For this review, take the finished solid that the model builds, in its own axes (mm). Face numbers are marked on the shaded views. A direction names the side the tool comes from. Give positions to 0.01 mm unless a question says otherwise; leave off trailing zeros. Order: outer loops, then holes, each group sorted by start corner. A loop starts at its lowest first (then second) coordinate and runs counter-clockwise, first axis right, second up. Notation, with made-up numbers: (22.25, 35.5) -> (56.25, 35.5) arc R24 cw to (56.25, 69.5) -> close; hole circle Ø4 at (73.25, 56.5). An arc over 180 degrees is marked (long way). Return JSON: item names as keys, results as strings. Group by question number.
1) The part is to be moulded in two halves that separate along X. For the marked faces 1, 2 and 3, say which applies: released by +X, released by -X, zero draft, split by the parting line, or undercut.
2) Add section C-C (x = -12). Give the boundary of the cut face in (y, z), then the cut area to 3 significant figures.
3) To check wall thickness, follow line 1 along X through (y, z) = (-17.5, -8); line 2 along X through (y, z) = (7, -7); line 3 along Z through (x, y) = (12.75, -5.05). State the ranges of each line that lie inside material, in increasing order.
4) Add section A-A (z = -21.5). Give the boundary of the cut face in (x, y).
5) For the marked faces 4, 5, 6 and 7, list the 3-axis set-ups (+Z, -Z, +X, -X, +Y, -Y) from which the entire face can be reached by the end or side of a thin tool; tool diameter is ignored.
6) Insertion check: P1, Ø2.5, axis at x = -7.525, y = -12.55, coming from the -Z side; P2, Ø10.5, axis at y = 1.5, z = -34.5, coming from the -X side; P3, Ø1.5, axis at x = 20, y = -18.5, coming from the -Z side. Each pin has a flat end and moves straight along its axis. Give the tip position at first contact, or say it passes through.
7) Add section D-D (x = -27.5). Give the boundary of the cut face in (y, z).
8) Add section B-B (y = -16.5). State how many separate pieces and enclosed holes the cut face has, then the cut area to 3 significant figures.
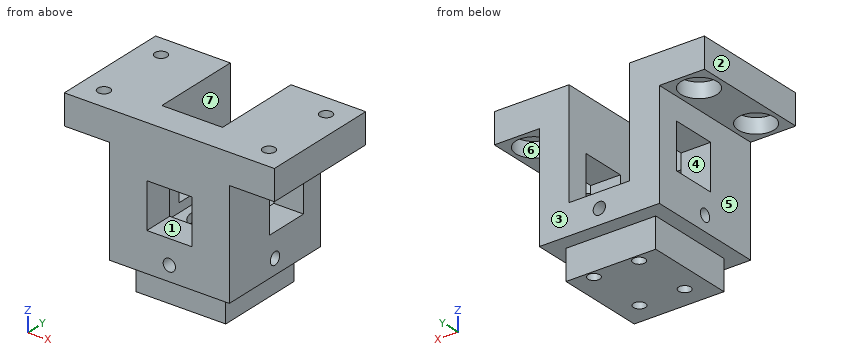
Autodesk Inventor part; units mm, degrees
ref_plane "YZ Plane" through (0, 0, 0) normal (1, 0, 0) x (0, 1, 0)
ref_plane "XZ Plane" through (0, 0, 0) normal (0, 1, 0) x (-1, 0, 0)
ref_plane "XY Plane" through (0, 0, 0) normal (0, 0, 1) x (1, 0, 0)
sketch "Sketch1" plane through (0, 0, 0) normal (0, 0, 1) x (1, 0, 0)
  line L0 (-20, -25.05) -> (20, -25.05)
  line L1 (20, -25.05) -> (20, 25.05)
  line L2 (20, 25.05) -> (-20, 25.05)
  line L3 (-20, 25.05) -> (-20, -25.05)
  line L4 (-20, -25.05) -> (20, 25.05) construction
  line L5 (20, -25.05) -> (-20, 25.05) construction
  point P0 (0, 0)
  dimension "d0" = 40
  dimension "d1" = 50.1
extrude "Extrusion1" add sketch "Sketch1" against normal blind 45.5
sketch "Sketch2" plane through (0, 0, 0) normal (0, 0, 1) x (1, 0, 0)
  line L0 (-10.1, -15.05) -> (10.1, -15.05)
  line L1 (10.1, -15.05) -> (10.1, 25.05)
  line L2 (10.1, 25.05) -> (-10.1, 25.05)
  line L3 (-10.1, 25.05) -> (-10.1, -15.05)
  line L4 (-10.1, -15.05) -> (10.1, 25.05) construction
  line L5 (10.1, -15.05) -> (-10.1, 25.05) construction
  line L6 (20, 25.05) -> (-20, 25.05)
  point P0 (0, 0)
  point P1 (0, 5)
  dimension "d4" = 20.2
  dimension "d5" = 40.1
extrude "Extrusion2" cut sketch "Sketch2" against normal blind 35.5
sketch "Sketch3" plane through (0, 0, -35.5) normal (0, 0, 1) x (1, 0, 0)
  circle A0 centre (0, -5.05) radius 7.5
  line L0 (10.1, -15.05) -> (-10.1, -15.05)
  point P0 (0, 0)
  dimension "d8" = 15
  dimension "d9" = 10
extrude "Extrusion3" cut sketch "Sketch3" against normal blind 6
sketch "Sketch4" plane through (0, 0, -45.5) normal (0, 0, -1) x (-1, 0, 0)
  line L0 (-14.95, -20) -> (14.95, -20)
  line L1 (14.95, -20) -> (14.95, 9.9)
  line L2 (14.95, 9.9) -> (-14.95, 9.9)
  line L3 (-14.95, 9.9) -> (-14.95, -20)
  line L4 (-14.95, -20) -> (14.95, 9.9) construction
  line L5 (14.95, -20) -> (-14.95, 9.9) construction
  line L6 (-20, -25.05) -> (20, -25.05)
  point P0 (0, 0)
  point P1 (0, -5.05)
  dimension "d12" = 29.9
  dimension "d13" = 29.9
  dimension "d14" = 20
extrude "Extrusion4" add sketch "Sketch4" along normal blind 10
sketch "Sketch5" plane through (20, -25.05, 0) normal (1, 0, 0) x (0, 0, -1)
  line L0 (17.5, 17.5) -> (32.5, 17.5)
  line L1 (32.5, 17.5) -> (32.5, 32.5)
  line L2 (32.5, 32.5) -> (17.5, 32.5)
  line L3 (17.5, 32.5) -> (17.5, 17.5)
  line L4 (17.5, 17.5) -> (32.5, 32.5) construction
  line L5 (32.5, 17.5) -> (17.5, 32.5) construction
  line L6 (45.5, 50.1) -> (45.5, 0)
  line L7 (0, 0) -> (45.5, 0)
  point P0 (0, 25.05)
  point P1 (25, 25)
  dimension "d17" = 15
  dimension "d18" = 15
  dimension "d19" = 13
  dimension "d20" = 17.5
extrude "Extrusion5" cut sketch "Sketch5" against normal through all
sketch "Sketch6" plane through (-20, -25.05, 0) normal (0, -1, 0) x (1, 0, 0)
  line L0 (27.5, -17.5) -> (12.5, -17.5)
  line L1 (12.5, -17.5) -> (12.5, -32.5)
  line L2 (12.5, -32.5) -> (27.5, -32.5)
  line L3 (27.5, -32.5) -> (27.5, -17.5)
  line L4 (27.5, -17.5) -> (12.5, -32.5) construction
  line L5 (12.5, -17.5) -> (27.5, -32.5) construction
  line L6 (40, -45.5) -> (0, -45.5)
  point P0 (20, 0)
  point P1 (20, -25)
  dimension "d23" = 15
  dimension "d24" = 15
  dimension "d25" = 13
extrude "Extrusion6" cut sketch "Sketch6" against normal through all
sketch "Sketch7" plane through (-20, 25.05, -45.5) normal (0, 1, 0) x (1, 0, 0)
  line L0 (0, -91) -> (40, -91)
  line L1 (40, -91) -> (40, 0)
  line L2 (40, 0) -> (0, 0)
  line L3 (0, 0) -> (0, -91)
  line L4 (0, -91) -> (40, 0) construction
  line L5 (40, -91) -> (0, 0) construction
  line L6 (0, 0) -> (40, 0)
  line L7 (40, -45.5) -> (40, 0)
  point P0 (20, -45.5)
extrude "Extrusion7" cut sketch "Sketch7" against normal blind 10.1
sketch "Sketch8" plane through (20, -25.05, 0) normal (1, 0, 0) x (0, 0, -1)
  line L0 (0, 0) -> (10, 0)
  line L1 (10, 0) -> (10, 40)
  line L2 (10, 40) -> (0, 40)
  line L3 (0, 40) -> (0, 0)
  line L4 (0, 0) -> (10, 40) construction
  line L5 (10, 0) -> (0, 40) construction
  line L6 (45.5, 40) -> (0, 40)
  line L7 (0, 0) -> (45.5, 0)
  line L8 (0, 0) -> (0, 40)
  point P0 (0, 25.05)
  point P1 (5, 20)
  dimension "d30" = 10
extrude "Extrusion8" add sketch "Sketch8" along normal blind 15
mirror "Mirror1" about plane through (0, 0, 0) normal (1, 0, 0) of "Extrusion8"
sketch "Sketch9" plane through (0, 0, 0) normal (0, 0, 1) x (1, 0, 0)
  circle A0 centre (27.5, 7.45) radius 2.05
  circle A1 centre (27.5, -17.55) radius 2.05
  circle A2 centre (-27.5, 7.45) radius 2.05
  circle A3 centre (-27.5, -17.55) radius 2.05
  line L0 (35, 14.95) -> (10.1, 14.95)
  line L1 (35, 14.95) -> (35, -25.05)
  line L2 (-35, -25.05) -> (35, -25.05)
  line L3 (-35, 14.95) -> (-35, -25.05)
  line L4 (-10.1, 14.95) -> (-35, 14.95)
  point P0 (0, 0)
  dimension "d33" = 4.1
  dimension "d34" = 4.1
  dimension "d35" = 4.1
  dimension "d36" = 4.1
  dimension "d37" = 7.5
  dimension "d38" = 7.5
  dimension "d39" = 7.5
  dimension "d40" = 7.5
  dimension "d41" = 7.5
  dimension "d42" = 7.5
  dimension "d43" = 7.5
  dimension "d44" = 7.5
extrude "Extrusion9" cut sketch "Sketch9" against normal through all
sketch "Sketch10" plane through (20, -25.05, -10) normal (0, 0, -1) x (-1, 0, 0)
  circle A0 centre (-7.5, 32.5) radius 2.05
  circle A1 centre (-7.5, 7.5) radius 2.05
  circle A2 centre (47.5, 32.5) radius 2.05
  circle A3 centre (47.5, 7.5) radius 2.05
  circle A4 centre (-7.5, 32.5) radius 6
  circle A5 centre (47.5, 32.5) radius 6
  circle A6 centre (47.5, 7.5) radius 6
  circle A7 centre (-7.5, 7.5) radius 6
  point P0 (20, 25.05)
  dimension "d47" = 12
  dimension "d48" = 12
  dimension "d49" = 12
  dimension "d50" = 12
extrude "Extrusion10" cut sketch "Sketch10" against normal blind 5
sketch "Sketch11" plane through (0, 0, -55.5) normal (0, 0, -1) x (-1, 0, 0)
  ellipse E0 centre (-7.952, -12.932) end of major axis (-8.818, -13.798) minor radius 1 (-9.07, -13.1556) -> (-8.1756, -14.05) ccw
  line L0 (8.1756, -14.05) -> (-8.1756, -14.05)
  ellipse E1 centre (7.952, -12.932) end of major axis (8.818, -13.798) minor radius 1 (8.1756, -14.05) -> (9.07, -13.1556) ccw
  line L1 (9.07, 23.1556) -> (9.07, -13.1556)
  ellipse E2 centre (7.952, 22.932) end of major axis (8.818, 23.798) minor radius 1 (9.07, 23.1556) -> (8.1756, 24.05) ccw
  line L2 (-8.1756, 24.05) -> (8.1756, 24.05)
  ellipse E3 centre (-7.952, 22.932) end of major axis (-8.818, 23.798) minor radius 1 (-8.1756, 24.05) -> (-9.07, 23.1556) ccw
  line L3 (-9.07, -13.1556) -> (-9.07, 23.1556)
  circle A0 centre (7.525, 22.55) radius 0.7835
  circle A1 centre (-7.525, 22.55) radius 0.7835
  circle A2 centre (7.525, 7.45) radius 0.7835
  circle A3 centre (-7.525, 7.45) radius 0.7835
  circle A4 centre (7.525, -12.55) radius 0.7835
  circle A5 centre (-7.525, -12.55) radius 0.7835
  circle A6 centre (0, -5.05) radius 6.4
  point P0 (0, 0)
hole "Hole1" at (-7.525, 7.45, -55.5) at (-7.525, -12.55, -55.5) at (7.525, 7.45, -55.5) at (7.525, -12.55, -55.5) direction (0, 0, 1) diameter 2.1 end through all
sketch "Sketch12" plane through (0, 0, -55.5) normal (0, 0, -1) x (-1, 0, 0)
  circle A0 centre (7.525, 7.45) radius 1.05
  circle A1 centre (7.525, -12.55) radius 1.05
  circle A2 centre (-7.525, -12.55) radius 1.05
  circle A3 centre (-7.525, 7.45) radius 1.05
  circle A4 centre (7.525, 7.45) radius 2
  circle A5 centre (7.525, -12.55) radius 2
  circle A6 centre (-7.525, -12.55) radius 2
  circle A7 centre (-7.525, 7.45) radius 2
  point P0 (0, 0)
  dimension "d60" = 4
  dimension "d61" = 4
  dimension "d62" = 4
  dimension "d63" = 4
extrude "Extrusion11" cut sketch "Sketch12" against normal blind 15 contours A0 | A1 | A2 | A3 | A4 | A5 | A6 | A7
sketch "Sketch13" plane through (20, -25.05, -45.5) normal (1, 0, 0) x (0, 0, -1)
  circle A0 centre (-5, 20) radius 2.05
  line L0 (-35.5, 0) -> (0, 0)
  line L1 (0, 40) -> (0, 0)
  point P0 (-45.5, 25.05)
  dimension "d66" = 4.1
  dimension "d67" = 20
  dimension "d68" = 5
extrude "Extrusion12" cut sketch "Sketch13" against normal through all
sketch "Sketch14" plane through (-20, 14.95, -45.5) normal (0, 1, 0) x (1, 0, 0)
  circle A0 centre (20, -5) radius 2.05
  line L0 (0, 0) -> (40, 0)
  point P0 (20, -45.5)
  dimension "d71" = 4.1
  dimension "d72" = 5
extrude "Extrusion13" cut sketch "Sketch14" against normal through all
properties part number "motor_bracket3" material "ABS Plastic"
Evaluation:
{
 "1": {"face 1": "undercut", "face 2": "released by -X", "face 3": "zero draft"},
 "2": {"outline": "(-25.05, -45.5) -> (-20, -45.5) -> (-20, -55.5) -> (9.9, -55.5) -> (9.9, -45.5) -> (14.95, -45.5) -> (14.95, 0) -> (-25.05, 0) -> close; hole (-7.55, -32.5) -> (7.45, -32.5) -> (7.45, -17.5) -> (-7.55, -17.5) -> close; hole circle Ø4.1 at (-5.05, -40.5)", "area": "1,880 mm^2"},
 "3": {"line 1": "-35 to -33.5, -21.5 to 21.5, 33.5 to 35", "line 2": "-35 to -33.48, -21.52 to -10.1, 10.1 to 21.52, 33.48 to 35", "line 3": "-55.5 to -42.55, -38.45 to -32.5, -17.5 to 0"},
 "4": {"outline": "(-20, -25.05) -> (-7.5, -25.05) -> (-7.5, -15.05) -> (-10.1, -15.05) -> (-10.1, -7.55) -> (-20, -7.55) -> close; (-20, 7.45) -> (-10.1, 7.45) -> (-10.1, 14.95) -> (-20, 14.95) -> close; (7.5, -25.05) -> (20, -25.05) -> (20, -7.55) -> (10.1, -7.55) -> (10.1, -15.05) -> (7.5, -15.05) -> close; (10.1, 7.45) -> (20, 7.45) -> (20, 14.95) -> (10.1, 14.95) -> close"},
 "5": {"face 4": "+X, -X", "face 5": "-Z, -X, +Y, -Y", "face 6": "-Z", "face 7": "+Z, +Y"},
 "6": {"P1": "z = -40.5", "P2": "x = -20", "P3": "z = -45.5"},
 "7": {"outline": "(-25.05, -10) -> (-23.55, -10) -> (-23.55, -5) -> (-19.6, -5) -> (-19.6, 0) -> (-25.05, 0) -> close; (-15.5, -5) -> (-11.55, -5) -> (-11.55, -10) -> (1.45, -10) -> (1.45, -5) -> (5.4, -5) -> (5.4, 0) -> (-15.5, 0) -> close; (9.5, -5) -> (13.45, -5) -> (13.45, -10) -> (14.95, -10) -> (14.95, 0) -> (9.5, 0) -> close"},
 "8": {"separate pieces": "3", "enclosed holes": "2", "area": "2,030 mm^2"}
}
